The listing builds one solid part. Answer for the finished solid, in the listing's coordinates (mm). A direction names the side the tool comes from. Round coordinates to 2 decimals unless told otherwise and drop trailing zeros. Order: outer loops, then holes, each group sorted by start corner. A loop starts at its lowest first (then second) coordinate and runs counter-clockwise, first axis right, second up. Notation, with made-up numbers: M -17.5,-1.5 L 27.5,-1.5 A13 cw 27.5,8.5 Z; hole C 10,-27 d6. An arc over 180 degrees is marked long. Put each result on its own line as item: value. Start each with the question number.
1. The part is cut by section C-C (y = -5). Give the vertices of the cut face in (x, z) (3 decimals), then the cut area to 3 significant figures.
2. Which of the six approach directions +Z, -Z, +X, -X, +Y, -Y give full straight-line access (tool end or side, diameter ignored) to faces 1 (the face through (-2.19, -17.12, 16.7)), 2 (the face through (-0.41, -7.51, -1.86))?
3. Consider line 1 (Z direction, x = 0, y = -6.75) (3 decimals); line 2 (Z direction, x = 0, y = -21.25) (3 decimals); line 3 (Y direction, x = -5, z = 15.5). Determine where each line is inside the solid, lowest interval first.
4. The mould has two halves that part along X. Classify faces 3 (the face through (-6.883, -12.522, -30.995)), 4 (the face through (-3, -19.05, 17)), 5 (the face through (-22, -25.4, -7)): +X half, -X half, draft (parallel to the pull), parting line (faces both ways), or undercut.
5. Each of these flat-tipped pins is pushed along its axis until it touches: pin 1 Ø4 at (y, z) = (-9, -17) entering from -X; pin 2 Ø10 at (x, y) = (-7.5, -14.5) entering from -Z; pin 3 Ø1 at (y, z) = (-8, -18) entering from -X. Where does it stop, or does it pass through?
6. The part is cut by section B-B (z = 0). Give the vertices of the cut face in (x, y) (3 decimals), then the cut area to 3 significant figures.
7. The part is cut by section D-D (x = -18.5). Give the vertices of the cut face in (y, z).
8. The part is cut by section A-A (x = 0). Give the vertices of the cut face in (y, z) (3 decimals), then the cut area to 3 significant figures.
from build123d import *

# Parameters (mm, degrees)
F0_R     = 22.225
F0_R_2   = 16.8413804611
F1_DEPTH = 19.05
F0_R_3   = 31.75
F2_DEPTH = 25.4
F0_R_4   = 1.905
F4_DEPTH = 15.24


# Not quite as in the source:
# - the program builds the solid bodies; features that only make, move or delete a surface that nothing else refers to are left out


with BuildPart() as f1:
    # F0 (on Front) → F1 (new body)
    with BuildSketch(Plane.XZ):
        Circle(F0_R)
        Circle(F0_R_2, mode=Mode.SUBTRACT)
    extrude(amount=F1_DEPTH)

    # F0 (on Front) → F2 (join)
    with BuildSketch(Plane.XZ):
        Circle(F0_R_3)
        Circle(F0_R, mode=Mode.SUBTRACT)
    extrude(amount=F2_DEPTH)

    # F0 (on Front) → F4 (join)
    with BuildSketch(Plane.XZ):
        Circle(F0_R_2)
        Circle(F0_R_4, mode=Mode.SUBTRACT)
    extrude(amount=F4_DEPTH)


solid = f1.part
Resolved:
1. outline: C 0,0 d63.5; hole C 0,0 d3.81
1. area: 3,160 mm2
2. face 1: -Y
2. face 2: +Y, -Y
3. line 1: -31.75 to -1.905, 1.905 to 31.75
3. line 2: -31.75 to -22.225, 22.225 to 31.75
3. line 3: -15.24 to 0
4. face 3: parting line
4. face 4: undercut
4. face 5: draft
5. pin 1: x = -27.98
5. pin 2: z = -31.65
5. pin 3: x = -26.49
6. outline: M -31.75,-25.4 L -22.225,-25.4 L -22.225,-19.05 L -16.841,-19.05 L -16.841,-15.24 L -1.905,-15.24 L -1.905,0 L -31.75,0 Z; M 1.905,-15.24 L 16.841,-15.24 L 16.841,-19.05 L 22.225,-19.05 L 22.225,-25.4 L 31.75,-25.4 L 31.75,0 L 1.905,0 Z
6. area: 1,140 mm2
7. outline: M -25.4,-25.8 L 0,-25.8 L 0,25.8 L -25.4,25.8 L -25.4,12.32 L -19.05,12.32 L -19.05,-12.32 L -25.4,-12.32 Z
8. outline: M -25.4,-31.75 L 0,-31.75 L 0,-1.905 L -15.24,-1.905 L -15.24,-16.841 L -19.05,-16.841 L -19.05,-22.225 L -25.4,-22.225 Z; M -25.4,22.225 L -19.05,22.225 L -19.05,16.841 L -15.24,16.841 L -15.24,1.905 L 0,1.905 L 0,31.75 L -25.4,31.75 Z
8. area: 1,140 mm2
